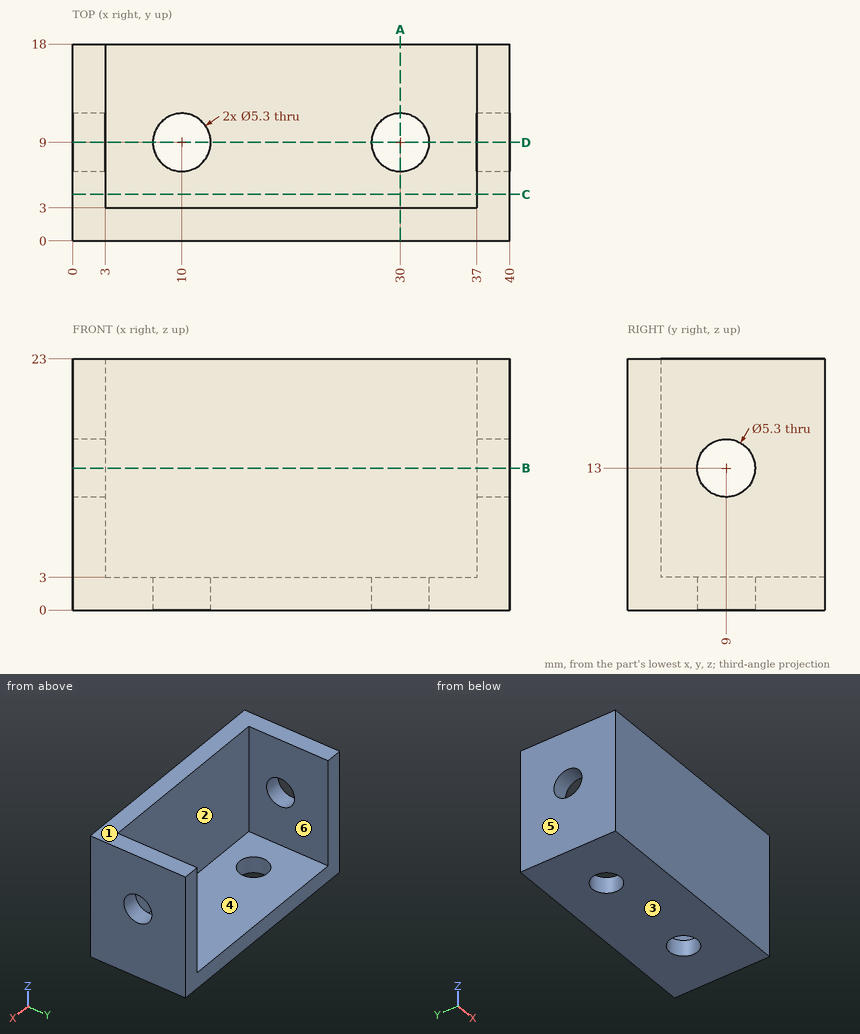
Study the drawing (mm; zero at the part's minimum x, y, z) and answer. A direction names the side the tool comes from. Give positions to 0.01 mm unless a question says otherwise; leave off trailing zeros. Order: outer loops, then holes, each group sorted by start corner. A loop starts at its lowest first (then second) coordinate and runs counter-clockwise, first axis right, second up.
1) Find section D-D on y = 9. Write down the section's boundary in (x, z), then the cut area to 3 significant figures.
Reported:
outline: (0, 0) - (7.35, 0) - (7.35, 3) - (3, 3) - (3, 10.35) - (0, 10.35) - close; (0, 15.65) - (3, 15.65) - (3, 23) - (0, 23) - close; (12.65, 0) - (27.35, 0) - (27.35, 3) - (12.65, 3) - close; (32.65, 0) - (40, 0) - (40, 10.35) - (37, 10.35) - (37, 3) - (32.65, 3) - close; (37, 15.65) - (40, 15.65) - (40, 23) - (37, 23) - close
area: 176 mm2
2) Given P1, Ø5, axis at x = 6.5, z = 9, coming from the +Y side; P2, Ø3, axis at y = 9, z = 13, coming from the -X side; P3, Ø7, axis at x = 10, y = 9, coming from the +Z side, each flat-ended and moving along its own axis, determine where each tip first touches the part or whether it passes through.
Reported:
P1: stops at y = 3
P2: passes through
P3: stops at z = 3
3) Find section C-C on y = 4.25. Write down the section's boundary in (x, z), then the cut area to 3 significant figures.
Reported:
outline: (0, 0) - (40, 0) - (40, 23) - (37, 23) - (37, 3) - (3, 3) - (3, 23) - (0, 23) - close
area: 240 mm2
4) Determine the mould class of the marked faces 3, 4, 5 and 6 for opening direction X: pulls with the +X half, pulls with the -X half, needs draft (parallel to the pull), parting line crosses it, or undercut.
Reported:
face 3: needs draft
face 4: undercut
face 5: pulls with the -X half
face 6: undercut
5) Find section B-B on z = 13. Write down the section's boundary in (x, y).
Reported:
outline: (0, 0) - (40, 0) - (40, 6.35) - (37, 6.35) - (37, 3) - (3, 3) - (3, 6.35) - (0, 6.35) - close; (0, 11.65) - (3, 11.65) - (3, 18) - (0, 18) - close; (37, 11.65) - (40, 11.65) - (40, 18) - (37, 18) - close
6) Find section A-A on x = 30. Write down the section's boundary in (y, z).
Reported:
outline: (0, 0) - (6.35, 0) - (6.35, 3) - (3, 3) - (3, 23) - (0, 23) - close; (11.65, 0) - (18, 0) - (18, 3) - (11.65, 3) - close
7) Consider line 1 along Y through (x, z) = (10, 2.2); line 2 along X through (y, z) = (12.75, 3.5); line 3 along Z through (x, y) = (0.7, 9). Determine where each line is inside the solid, lowest interval first.
Reported:
line 1: y = 0 to 6.35, 11.65 to 18
line 2: x = 0 to 3, 37 to 40
line 3: z = 0 to 10.35, 15.65 to 23
8) For the marked faces 1 and 2, determine the directions among +Z, -Z, +X, -X, +Y, -Y from which every point of the face is accessible in a straight line to the end or side of a thin tool.
Reported:
face 1: +Z, +X, -X, +Y, -Y
face 2: +Z, +Y
